Verification items for this drawing (mm, ordinates from the low corner). Round coordinates to 2 decimals unless told otherwise and drop trailing zeros. Write each loop counter-clockwise with the first axis right and the second up, starting at its lowest first coordinate (ties: lowest second). Pieces come first, ordered by that corner, then holes. Notation, with made-up numbers: (8.5, 73.25) -> (17.5, 73.25) arc R32 ccw to (17.5, 102.25) -> close; hole circle Ø1 at (80, 29). An arc over 180 degrees is marked (long way). One line per question, with ' | ' between items.
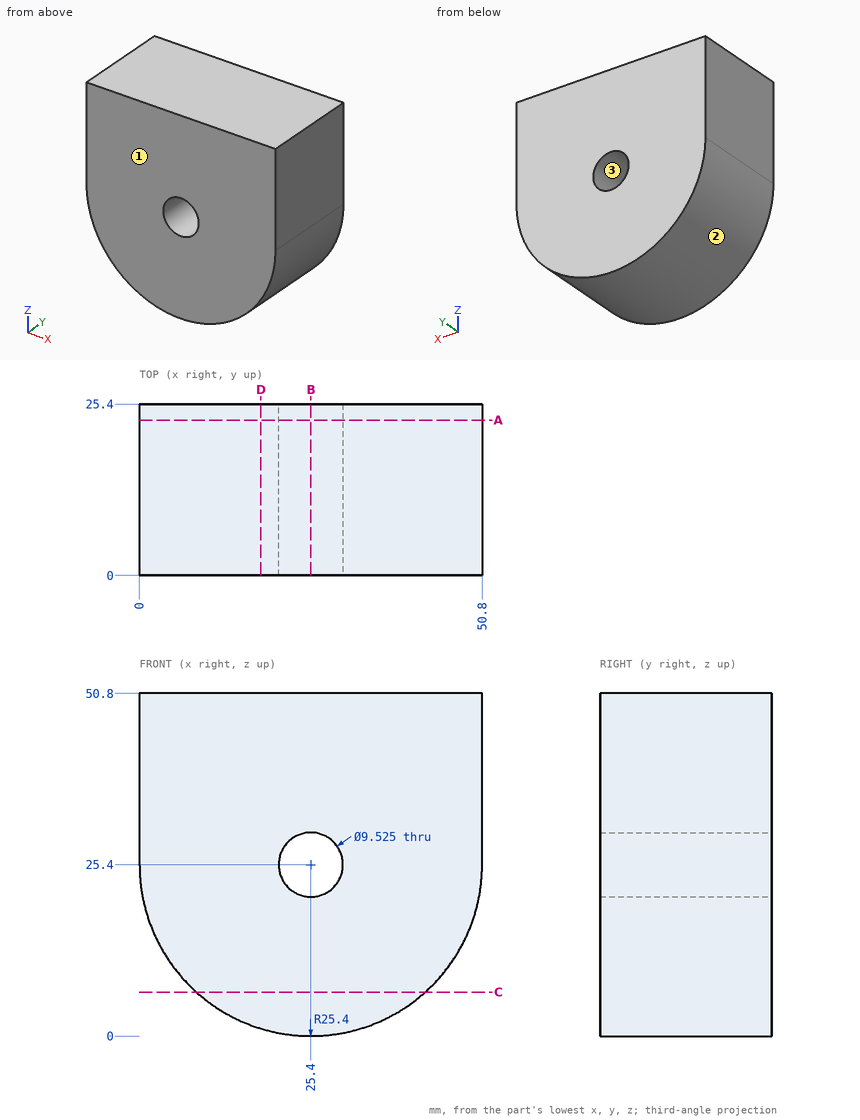
(1) Sectioned sample at A-A on y = 23. Record the cut outline in (x, z) (1 decimal).
Resolved:
outline: (0, 25.4) arc R25.4 ccw to (50.8, 25.4) -> (50.8, 50.8) -> (0, 50.8) -> close; hole circle Ø9.5 at (25.4, 25.4)
(2) Go/stop test with a flat-tipped pin: pin 1 (5 mm diameter, centred on y = 10.5, z = 12, fed in from -X). Record where the tip stops, or that it passes through.
Resolved:
pin 1: stops at x = 2.46
(3) Sectioned sample at D-D on x = 18. Record the cut outline in (y, z), then the cut area to 3 significant figures.
Resolved:
outline: (0, 1.1) -> (25.4, 1.1) -> (25.4, 50.8) -> (0, 50.8) -> close | area: 1,260 mm2
(4) Draft check along X on the marked faces 1, 2 and 3. Enter one of: +X half, -X half, draft (parallel to the pull), parting line (faces both ways), or undercut.
Resolved:
face 1: draft | face 2: parting line | face 3: undercut
(5) Sectioned sample at B-B on x = 25.4. Record the cut outline in (y, z).
Resolved:
outline: (0, 0) -> (25.4, 0) -> (25.4, 20.64) -> (0, 20.64) -> close; (0, 30.16) -> (25.4, 30.16) -> (25.4, 50.8) -> (0, 50.8) -> close
(6) Sectioned sample at C-C on z = 6.5. Record the cut outline in (x, y).
Resolved:
outline: (8.43, 0) -> (42.37, 0) -> (42.37, 25.4) -> (8.43, 25.4) -> close
(7) Material ranges on line 1 (Z direction, x = 25.4, y = 17.5); line 2 (X direction, y = 2.5, z = 26.5); line 3 (Z direction, x = 26, y = 10), recorded low to high.
Resolved:
line 1: z = 0 to 20.64, 30.16 to 50.8 | line 2: x = 0 to 20.77, 30.03 to 50.8 | line 3: z = 0.01 to 20.68, 30.12 to 50.8
